For this review, take the finished solid that the model builds, in its own axes (mm). Coordinates: 2 decimals unless noted, no trailing zeros. Write each loop counter-clockwise with the first axis right and the second up, starting at its lowest first coordinate (ties: lowest second). Pieces come first, ordered by that corner, then holes.
```python
from build123d import *

# Parameters (mm, degrees)
F0_W     = 528.32
F0_H     = 25.4
F1_DEPTH = 3.175
F2_W     = 502.92
F2_H     = 7.62
F3_DEPTH = 1.016
F4_R     = 1.8288
F5_DEPTH = 6.351
F7_D     = 2.2606
F8_R     = 2.54
F9_R     = 1.27


with BuildPart() as f1:
    # F0 (on Top) → F1 (new body, symmetric)
    with BuildSketch(Plane.XY):
        Rectangle(F0_W, F0_H)
    extrude(amount=F1_DEPTH, both=True)

    # F2 (on face) → F3 (cut)
    with BuildSketch(Plane.XY.offset(3.175)):
        with Locations((0, -1.27)):
            Rectangle(F2_W, F2_H)
    extrude(amount=-F3_DEPTH, mode=Mode.SUBTRACT)

    # F4 (on face) → F5 (cut, through all)
    with BuildSketch(Plane.XY.offset(3.175)):
        with Locations((-257.81, 0)):
            Circle(F4_R)
        with Locations((257.81, 0)):
            Circle(F4_R)
    extrude(amount=-F5_DEPTH, mode=Mode.SUBTRACT)

    # F7 (through all)
    with Locations(Plane.XY.offset(3.175)):
        with Locations((-60.96, -10.16), (-40.64, -10.16), (182.88, -10.16), (-121.92, -10.16), (-81.28, -10.16), (-101.6, -10.16), (203.2, -10.16), (60.96, -10.16), (40.64, -10.16), (243.84, -10.16), (223.52, -10.16), (-20.32, -10.16), (162.56, -10.16), (0, -10.16), (20.32, -10.16), (142.24, -10.16), (121.92, -10.16), (101.6, -10.16), (81.28, -10.16), (-243.84, -10.16), (-223.52, -10.16), (-203.2, -10.16), (-182.88, -10.16), (-162.56, -10.16), (-142.24, -10.16)):
            Hole(F7_D / 2)

    # F8
    f8_edges = [f1.edges().sort_by_distance(p)[0] for p in [
        (264.16, -12.7, 0),
        (264.16, 12.7, 0),
        (-264.16, -12.7, 0),
        (-264.16, 12.7, 0),
    ]]
    fillet(f8_edges, radius=F8_R)

    # F9
    f9_edges = [f1.edges().sort_by_distance(p)[0] for p in [
        (-251.46, -5.08, 2.667),
        (-251.46, 2.54, 2.667),
        (251.46, -5.08, 2.667),
        (251.46, 2.54, 2.667),
    ]]
    fillet(f9_edges, radius=F9_R)


solid = f1.part
```
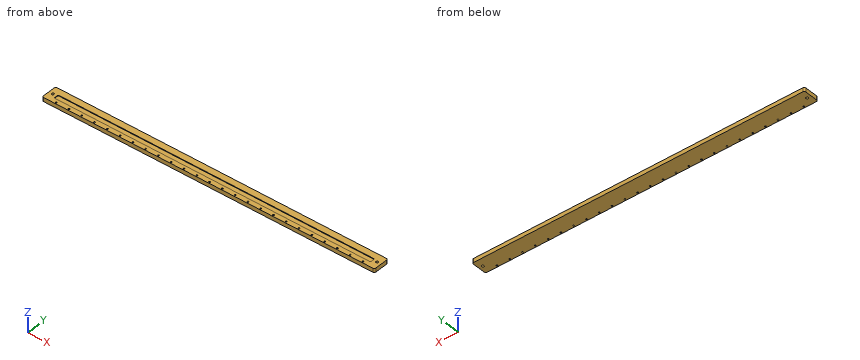
Q1. For probe 1 along X at (y, z) = (0.5, -1); probe 2 along Y at (x, z) = (30, 2.75); probe 3 along Z at (x, y) = (-178.5, 0.25) (3 decimals), list the stretches that pass through material, from the lowest coordinate up.
Ans:
probe 1: x = -264.16 to -259.57, -256.05 to 256.05, 259.57 to 264.16
probe 2: y = -12.7 to -5.08, 2.54 to 12.7
probe 3: z = -3.175 to 2.159
Q2. Add section A-A (x = -109.5). State the section outline as (y, z) points (3 decimals), then the cut area to 3 significant figures.
Ans:
outline: (-12.7, -3.175) - (12.7, -3.175) - (12.7, 3.175) - (2.54, 3.175) - (2.54, 2.159) - (-5.08, 2.159) - (-5.08, 3.175) - (-12.7, 3.175) - close
area: 154 mm2
Q3. Clearance check with a flat-ended pin moving along its axis: pin 1 Ø6 at (x, y) = (-59.5, -0.5) entering from +Z. State where the tip first meets the part, or that it passes through.
Ans:
pin 1: stops at z = 2.16
